from build123d import *

# Parameters (mm, degrees)
SKETCH_1_R          = 22.5
SKETCH_1_R_2        = 12.5
SKETCH_1_R_3        = 1.3
EXTRUDE_1_DEPTH     = 4
EXTRUDE_START       = -4
EXTRUDE_2_DEPTH     = 4
SKETCH_3_W          = 45
SKETCH_3_H          = 5
EXTRUDE_3_DEPTH     = 8
CUT_EXTRUDE_START   = -10
CUT_EXTRUDE_2_DEPTH = 10
SKETCH_6_R          = 1.3
SKETCH_6_R_2        = 12.5
EXTRUDE_4_DEPTH     = 8
CUT_EXTRUDE_3_DEPTH = 4
SKETCH_8_R          = 2.5
CUT_EXTRUDE_4_DEPTH = 10
SKETCH_9_W          = 45
SKETCH_9_H          = 5
EXTRUDE_5_DEPTH     = 10
FILLET_1_R          = 1
CUT_EXTRUDE_5_DEPTH = 3
SKETCH_11_R         = 1.65
CUT_EXTRUDE_6_DEPTH = 13


with BuildPart() as part:
    # 草图1 → 凸台-拉伸1 (new body)
    with BuildSketch(Plane.XY):
        Circle(SKETCH_1_R)
        Circle(SKETCH_1_R_2, mode=Mode.SUBTRACT)
        with Locations((0, 20)):
            Circle(SKETCH_1_R_3, mode=Mode.SUBTRACT)
        with Locations((-17.320508076, -10)):
            Circle(SKETCH_1_R_3, mode=Mode.SUBTRACT)
        with Locations((17.320508076, -10)):
            Circle(SKETCH_1_R_3, mode=Mode.SUBTRACT)
    extrude(amount=EXTRUDE_1_DEPTH)

    # 草图2 → 凸台-拉伸2 (add)
    with BuildSketch(Plane.XY.offset(4).offset(EXTRUDE_START)):
        with BuildLine():
            Line((-22.5, 0), (-22.5, -20))
            Line((-22.5, -20), (-10.307764064, -20))
            ThreePointArc((-10.307764064, -20), (-19.211646096, -11.711646096), (-22.5, 0))
        make_face()
        with BuildLine():
            Line((22.5, -20), (22.5, 0))
            ThreePointArc((22.5, 0), (19.211646096, -11.711646096), (10.307764064, -20))
            Line((10.307764064, -20), (22.5, -20))
        make_face()
    extrude(amount=EXTRUDE_2_DEPTH)

    # 草图3 → 凸台-拉伸3 (add)
    with BuildSketch(Plane.XY.offset(4)):
        with Locations((0, -17.5)):
            Rectangle(SKETCH_3_W, SKETCH_3_H)
    extrude(amount=EXTRUDE_3_DEPTH)

    # 草图5 → 切除-拉伸2 (cut)
    with BuildSketch(Plane.XY.offset(4).offset(CUT_EXTRUDE_START)):
        with BuildLine():
            Line((10.307764064, -20), (-10.307764064, -20))
            ThreePointArc((-10.307764064, -20), (0, -22.5), (10.307764064, -20))
        make_face()
    extrude(amount=CUT_EXTRUDE_2_DEPTH, mode=Mode.SUBTRACT)

    # 草图6 → 凸台-拉伸4 (add)
    with BuildSketch(Plane.XY.offset(4)):
        with BuildLine():
            Line((-22.5, -15), (22.5, -15))
            Line((22.5, -15), (22.5, 0))
            ThreePointArc((22.5, 0), (0, 22.5), (-22.5, 0))
            Line((-22.5, 0), (-22.5, -15))
        make_face()
        with Locations(Location((17.320508076, -10, 0), (0, 0, 180))):
            Circle(SKETCH_6_R, mode=Mode.SUBTRACT)
        with Locations(Location((-17.320508076, -10, 0), (0, 0, 180))):
            Circle(SKETCH_6_R, mode=Mode.SUBTRACT)
        with Locations(Location((0, 20, 0), (0, 0, 180))):
            Circle(SKETCH_6_R, mode=Mode.SUBTRACT)
        with Locations(Location((0, 0, 0), (0, 0, 180))):
            Circle(SKETCH_6_R_2, mode=Mode.SUBTRACT)
    extrude(amount=EXTRUDE_4_DEPTH)

    # 草图7 → 切除-拉伸3 (cut)
    with BuildSketch(Plane(origin=(0, 0, 0), x_dir=(-1, 0, 0), z_dir=(0, 0, -1))):
        with BuildLine():
            Line((-22.5, 0), (-22.5, -20))
            Line((-22.5, -20), (22.5, -20))
            Line((22.5, -20), (22.5, 0))
            ThreePointArc((22.5, 0), (0, 22.5), (-22.5, 0))
        make_face()
    extrude(amount=-CUT_EXTRUDE_3_DEPTH, mode=Mode.SUBTRACT)

    # 草图8 → 切除-拉伸4 (cut)
    with BuildSketch(Plane.XY.offset(12)):
        with Locations((14.071515431, 8.124193222)):
            Circle(SKETCH_8_R)
    extrude(amount=-CUT_EXTRUDE_4_DEPTH, mode=Mode.SUBTRACT)

    # 草图9 → 凸台-拉伸5 (add)
    with BuildSketch(Plane.XY.offset(12)):
        with Locations((0, -17.5)):
            Rectangle(SKETCH_9_W, SKETCH_9_H)
    extrude(amount=EXTRUDE_5_DEPTH)

    # 圆角1
    fillet_1_edges = [part.edges().sort_by_distance(p)[0] for p in [
        (0, -15, 12),
    ]]
    fillet(fillet_1_edges, radius=FILLET_1_R)

    # 草图10 → 切除-拉伸5 (cut)
    with BuildSketch(Plane(origin=(0, 0, 4), x_dir=(-1, 0, 0), z_dir=(0, 0, -1))):
        with BuildLine():
            Line((-22.5, 0), (-22.5, -20))
            Line((-22.5, -20), (22.5, -20))
            Line((22.5, -20), (22.5, 0))
            ThreePointArc((22.5, 0), (0, 22.5), (-22.5, 0))
        make_face()
    extrude(amount=-CUT_EXTRUDE_5_DEPTH, mode=Mode.SUBTRACT)

    # 草图11 → 切除-拉伸6 (cut)
    with BuildSketch(Plane(origin=(0, -15, 0), x_dir=(1, 0, 0), z_dir=(0, 1, 0))):
        with Locations(Location((-12.5, -17.5, 0), (0, 0, 270))):
            Circle(SKETCH_11_R)
        with Locations(Location((12.5, -17.5, 0), (0, 0, 270))):
            Circle(SKETCH_11_R)
    extrude(amount=-CUT_EXTRUDE_6_DEPTH, mode=Mode.SUBTRACT)


solid = part.part
Read the model definition and answer for the solid it produces. Units are mm, in the model's axes. A direction names the side the tool comes from. Round coordinates to 2 decimals unless told otherwise and drop trailing zeros. Order: outer loops, then holes, each group sorted by start corner. A loop starts at its lowest first (then second) coordinate and runs counter-clockwise, first axis right, second up.
1) Straight lines are drawn through the part: L1, parallel to X at y = -18.4, z = 17.5; L2, parallel to X at y = -10.5, z = 10.75; L3, parallel to Y at x = -9.5, z = 19.75. For each, find the intervals that lie inside material, in ascending order.
2) The mould has two halves that part along Z. Classify faces 3 (the face through (0, -17, 22)), 4 (the face through (-18.56, -10.39, 9.46)), 5 (the face through (-13.132, -17.465, 19.024)): released by +Z, released by -Z, zero draft, split by the parting line, or undercut.
3) For faces 1 (the face through (0, 13, 12)), 2 (the face through (-11.923, -3.755, 9.465)), determine the directions among +Z, -Z, +X, -X, +Y, -Y from which every point of the face is accessible in a straight line to the end or side of a thin tool.
4) The part is cut by section C-C on x = 0. Write down the section's boundary in (y, z), plus the area to 3 significant figures.
5) Flat-ended cylindrical pins translate along their axes: pin 1 (7 mm diameter, centred on x = 2, z = 16, fed in from +Y); pin 2 (1.5 mm diameter, centred on y = -12.5, z = 14, fed in from +X); pin 3 (5 mm diameter, centred on y = 5.5, z = 13, fed in from -X); pin 4 (6.5 mm diameter, centred on x = 14.07, y = 8.12, fed in from -Z). Find the tip coordinate at first contact, or state that the pin passes through.
6) The part is cut by section A-A on z = 17.5. Write down the section's boundary in (x, y).
7) The part is cut by section D-D on y = 6.5. Write down the section's boundary in (x, z), plus the area to 3 significant figures.
8) The part is cut by section B-B on y = -7. Write down the section's boundary in (x, z).
Resolved:
1. L1: x = -22.5 to -14.15, -10.85 to 10.85, 14.15 to 22.5
1. L2: x = -22.5 to -18.52, -16.12 to -6.78, 6.78 to 16.12, 18.52 to 22.5
1. L3: y = -20 to -15
2. face 3: released by +Z
2. face 4: zero draft
2. face 5: undercut
3. face 1: +Z, +X, -X, +Y
3. face 2: +Z, -Z
4. outline: (-20, 7) - (-12.5, 7) - (-12.5, 12) - (-14, 12) arc R1 cw to (-15, 13) - (-15, 22) - (-20, 22) - close; (12.5, 7) - (18.7, 7) - (18.7, 12) - (12.5, 12) - close; (21.3, 7) - (22.5, 7) - (22.5, 12) - (21.3, 12) - close
4. area: 125 mm2
5. pin 1: stops at y = -14.87
5. pin 2: passes through
5. pin 3: stops at x = -22.27
5. pin 4: stops at z = 7
6. outline: (-22.5, -20) - (-14.15, -20) - (-14.15, -15) - (-22.5, -15) - close; (-10.85, -20) - (10.85, -20) - (10.85, -15) - (-10.85, -15) - close; (14.15, -20) - (22.5, -20) - (22.5, -15) - (14.15, -15) - close
7. outline: (-21.54, 7) - (-10.68, 7) - (-10.68, 12) - (-21.54, 12) - close; (10.68, 7) - (12.17, 7) - (12.17, 12) - (10.68, 12) - close; (15.97, 7) - (21.54, 7) - (21.54, 12) - (15.97, 12) - close
7. area: 89.6 mm2
8. outline: (-22.5, 7) - (-10.36, 7) - (-10.36, 12) - (-22.5, 12) - close; (10.36, 7) - (22.5, 7) - (22.5, 12) - (10.36, 12) - close
